Can you work these out from the model? Positions are in its coordinate system, mm. Face numbers are marked on the shaded views. Give positions to 0.01 mm unless a question says otherwise; leave off trailing zeros. Order: outer loops, then holes, each group sorted by start corner. A loop starts at its lowest first (then second) coordinate and runs counter-clockwise, first axis right, second up. Notation, with made-up numbers: (84.25, -3) -> (120.25, -3) arc R22 cw to (120.25, 35) -> close; hole circle Ø2 at (1.25, 66.5). An arc over 180 degrees is marked (long way). Answer as a JSON object with one key per item and string values.
```python
from build123d import *

# Parameters (mm, degrees)
SKETCH_1_R          = 7
EXTRUDE_1_DEPTH     = 2
SKETCH_2_R          = 4.25
EXTRUDE_2_DEPTH     = 6.8
CUT_EXTRUDE_1_REACH = 15.245
SKETCH_3_R          = 3.15
FILLET_1_R          = 0.5


with BuildPart() as part:
    # 草图1 → 凸台-拉伸1 (new body)
    with BuildSketch(Plane(origin=(0, 0, 0), x_dir=(1, 0, 0), z_dir=(0, 1, 0))):
        with Locations(Location((0, 0, 0), (0, 0, 270))):
            Circle(SKETCH_1_R)
    extrude(amount=EXTRUDE_1_DEPTH)

    # 草图2 → 凸台-拉伸2 (add)
    with BuildSketch(Plane(origin=(0, 2, 0), x_dir=(1, 0, 0), z_dir=(0, 1, 0))):
        with Locations(Location((0, 0, 0), (0, 0, 270))):
            Circle(SKETCH_2_R)
    extrude(amount=EXTRUDE_2_DEPTH)

    # 草图3 → 切除-拉伸1 (cut, up to next)
    with BuildSketch(Plane(origin=(0, 8.8, 0), x_dir=(1, 0, 0), z_dir=(0, 1, 0)), mode=Mode.PRIVATE) as cut_extrude_1_sk1:
        with Locations(Location((0, 0, 0), (0, 0, 270))):
            Circle(SKETCH_3_R)
    cut_extrude_1_tool1 = extrude(cut_extrude_1_sk1.sketch, amount=-CUT_EXTRUDE_1_REACH, mode=Mode.PRIVATE) & part.part
    add(cut_extrude_1_tool1.solids().sort_by_distance((0, 8.8, 0))[0], mode=Mode.SUBTRACT)

    # 圆角1
    fillet_1_edges = [part.edges().sort_by_distance(p)[0] for p in [
        (0, 2, -4.25),
    ]]
    fillet(fillet_1_edges, radius=FILLET_1_R)


solid = part.part
```
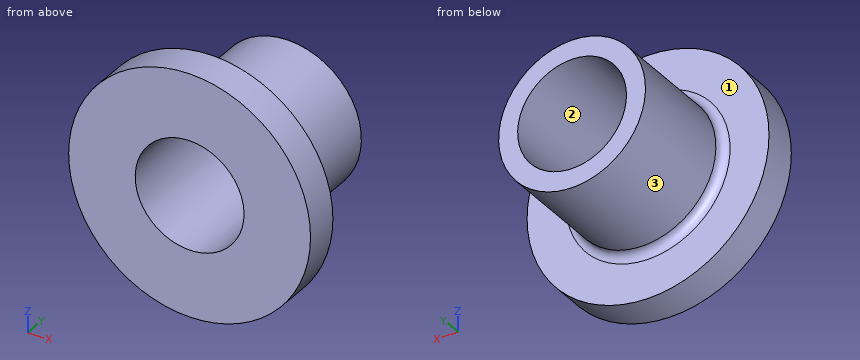
1. Please list where these lines run through material, in increasing order: L1, parallel to X at y = 4.5, z = 0; L2, parallel to Y at x = 3, z = 5; L3, parallel to X at y = 2.25, z = 0.
Worked answers:
{"L1": "-4.25 to -3.15, 3.15 to 4.25", "L2": "0 to 2", "L3": "-4.32 to -3.15, 3.15 to 4.32"}
2. If we section it at B-B on x = 0: Please give me the cut outline in (y, z), then the cut area to 3 significant figures.
Worked answers:
{"outline": "(0, -7) -> (2, -7) -> (2, -4.75) arc R0.5 cw to (2.5, -4.25) -> (8.8, -4.25) -> (8.8, -3.15) -> (0, -3.15) -> close; (0, 3.15) -> (8.8, 3.15) -> (8.8, 4.25) -> (2.5, 4.25) arc R0.5 cw to (2, 4.75) -> (2, 7) -> (0, 7) -> close", "area": "30.5 mm²"}
3. Will these pins go through, and if not, where does the flat tip stop? pin 1 Ø3 at (x, y) = (4, 7) entering from -Z; pin 2 Ø3 at (x, y) = (1.5, 6.5) entering from +Z; pin 3 Ø3 at (x, y) = (3, 7) entering from +Z.
Worked answers:
{"pin 1": "z = -3.44", "pin 2": "z = 4.25", "pin 3": "z = 3.98"}
4. If we mould it in two halves opening along Z, with no side actions, what happens to the marked faces 1, 2 and 3? For each: +Z half, -Z half, draft (parallel to the pull), parting line (faces both ways), or undercut.
Worked answers:
{"face 1": "draft", "face 2": "undercut", "face 3": "parting line"}
5. If we section it at A-A on z = 0: Please give me the cut outline in (x, y), then the cut area to 3 significant figures.
Worked answers:
{"outline": "(-7, 0) -> (-3.15, 0) -> (-3.15, 8.8) -> (-4.25, 8.8) -> (-4.25, 2.5) arc R0.5 cw to (-4.75, 2) -> (-7, 2) -> close; (3.15, 0) -> (7, 0) -> (7, 2) -> (4.75, 2) arc R0.5 cw to (4.25, 2.5) -> (4.25, 8.8) -> (3.15, 8.8) -> close", "area": "30.5 mm²"}
6. If we section it at D-D on y = 6.5: Please give me the cut outline in (x, z), then the cut area to 3 significant figures.
Worked answers:
{"outline": "circle Ø8.5 at (0, 0); hole circle Ø6.3 at (0, 0)", "area": "25.6 mm²"}
7. If we section it at C-C on y = 1.5: Please give me the cut outline in (x, z).
Worked answers:
{"outline": "circle Ø14 at (0, 0); hole circle Ø6.3 at (0, 0)"}
